Verification items for the finished model (mm, model axes). A direction names the side the tool comes from. Round coordinates to 2 decimals unless told otherwise and drop trailing zeros. Loops run counter-clockwise (first coordinate to the right, second up) from the corner with the lowest first, then second, coordinate; pieces in that order, holes last. Notation, with made-up numbers: (20, 23) -> (28, 23) arc R21 cw to (28, 53) -> close; hole circle Ø3 at (62.5, 19.25). An arc over 180 degrees is marked (long way). Write item = value, one per line.
```python
from build123d import *

# Parameters (mm, degrees)
SKETCH_1_R                = 33
SKETCH_1_R_2              = 25
EXTRUDE_1_DEPTH           = 8
SKETCH_3_W                = 6
SKETCH_3_H                = 75.065219084
CUT_EXTRUDE_1_DEPTH       = 4
CUT_EXTRUDE_1_DRAFT       = -1
HOLE_WIZARD_1_D           = 10
HOLE_WIZARD_1_CBORE_D     = 15.2
HOLE_WIZARD_1_CBORE_DEPTH = 4


with BuildPart() as part:
    # 草图1 → 凸台-拉伸1 (new body)
    # profile 1 of 2: a face of its own
    with BuildSketch(Plane.XY):
        Circle(SKETCH_1_R)
        Circle(SKETCH_1_R_2, mode=Mode.SUBTRACT)
    # profile 2 of 2: a face of its own
    with BuildSketch(Plane.XY):
        with BuildLine():
            Line((39.646094734, 37.429095265), (-3.509900495, 32.8128115))
            ThreePointArc((-3.509900495, 32.8128115), (22.058708979, 24.544110458), (33, 0))
            ThreePointArc((33, 0), (28.248342415, -17.059635132), (15.361748435, -29.206449374))
            ThreePointArc((15.361748435, -29.206449374), (23.844645568, -28.056684557), (31.078097518, -32.63474919))
            ThreePointArc((31.078097518, -32.63474919), (37.364061613, -36.96690321), (44.997122438, -36.835428905))
            Line((44.997122438, -36.835428905), (71, -28))
            Line((71, -28), (71, 28))
            Line((71, 28), (44.997122438, 36.835428905))
            ThreePointArc((44.997122438, 36.835428905), (42.353950178, 37.42377389), (39.646094734, 37.429095265))
        make_face()
    extrude(amount=EXTRUDE_1_DEPTH)


with BuildPart() as cut_extrude_1_tool:
    # 草图3 → 切除-拉伸-薄壁1 (with draft: the straight prism first)
    with BuildSketch(Plane(origin=(0, 0, 0), x_dir=(-1, 0, 0), z_dir=(0, 0, -1))):
        with Locations((0, -0.589324586)):
            Rectangle(SKETCH_3_W, SKETCH_3_H)
    extrude(amount=-CUT_EXTRUDE_1_DEPTH)
    # 切除-拉伸-薄壁1: the draft: its side faces are tilted about the plane it starts from
    cut_extrude_1_sides = [cut_extrude_1_tool.faces().sort_by_distance(p)[0] for p in [
        (3, -0.589324586, 2),
        (0, -38.121934128, 2),
        (-3, -0.589324586, 2),
        (0, 36.943284956, 2),
    ]]
    draft(cut_extrude_1_sides, Plane(origin=(0, 0, 0), x_dir=(-1, 0, 0), z_dir=(0, 0, -1)), CUT_EXTRUDE_1_DRAFT)


with BuildPart() as part_1:
    add(part.part)

    # 切除-拉伸-薄壁1: cut by cut_extrude_1_tool
    add(cut_extrude_1_tool.part, mode=Mode.SUBTRACT)

    # 孔1 (through all)
    with Locations(Plane.XY.offset(8)):
        with Locations((40.975602497, 25), (40.975602497, -25)):
            CounterBoreHole(HOLE_WIZARD_1_D / 2, HOLE_WIZARD_1_CBORE_D / 2, HOLE_WIZARD_1_CBORE_DEPTH)


solid = part_1.part
```
(1) Sectioned sample at D-D, the plane x = 56. Record the cut outline in (y, z), and give its area (3 significant figures).
Filled sheet:
outline = (-33.1, 0) -> (33.1, 0) -> (33.1, 8) -> (-33.1, 8) -> close
area = 530 mm2
(2) Go/stop test with flat-tipped pins: pin 1 Ø4 at (x, z) = (43.5, 1) entering from +Y; pin 2 Ø13.5 at (x, y) = (40.98, -25) entering from +Z; pin 3 Ø3 at (x, y) = (0.5, -30.5) entering from -Z. Record where each tip stops, or that it passes through.
Filled sheet:
pin_1 = 37.49
pin_2 = 4
pin_3 = 4
(3) Material ranges on probe 1 along X at (y, z) = (0, 3.25); probe 2 along Y at (x, z) = (38.5, 5.5); probe 3 along X at (y, z) = (-26, 3), recorded low to high. Write a range as from..to.
Filled sheet:
probe_1 = -33..-25, 25..71
probe_2 = -37.25..-32.19, -17.81..17.81, 32.19..37.31
probe_3 = -20.32..-2.95, 2.95..36.08, 45.87..71
(4) Draft check along X on faces 3 (the face through (0, -29, 4)), 4 (the face through (58.181, 32.356, 3.944)), 5 (the face through (18.37, 35.153, 3.944)), 6 (the face through (-26, -2, 0)). Enter one of: released by +X, released by -X, zero draft, split by the parting line, or undercut.
Filled sheet:
face_3 = undercut
face_4 = released by +X
face_5 = released by -X
face_6 = zero draft
(5) Set-up check for faces 1 (the face through (45.06, 31.41, 6.03)), 2 (the face through (44, 1, 0)): record each of +Z, -Z, +X, -X, +Y, -Y from which the full face is reachable in a straight line by a thin tool's end or side.
Filled sheet:
face_1 = +Z
face_2 = -Z, +X, -X, +Y, -Y
(6) Sectioned sample at B-B, the plane y = 0. Record the cut outline in (x, z).
Filled sheet:
outline = (-33, 0) -> (-25, 0) -> (-25, 8) -> (-33, 8) -> close; (25, 0) -> (71, 0) -> (71, 8) -> (25, 8) -> close
(7) Sectioned sample at A-A, the plane z = 2.5. Record the cut outline in (x, y), and give its area (3 significant figures).
Filled sheet:
outline = (-3.51, 32.81) arc R33 ccw to (-2.96, -32.87) -> (-2.96, -24.82) arc R25 cw to (-2.96, 24.82) -> (-2.96, 32.87) -> close; (2.96, -32.87) arc R33 ccw to (15.36, -29.21) arc R12.5 cw to (31.08, -32.63) arc R12.5 ccw to (45, -36.84) -> (71, -28) -> (71, 28) -> (45, 36.84) arc R12.5 ccw to (39.65, 37.43) -> (2.96, 33.5) -> (2.96, 24.82) arc R25 cw to (2.96, -24.82) -> close; hole circle Ø10 at (40.98, -25); hole circle Ø10 at (40.98, 25)
area = 4,230 mm2
(8) Sectioned sample at C-C, the plane x = 0. Record the cut outline in (y, z).
Filled sheet:
outline = (-33, 4) -> (-25, 4) -> (-25, 8) -> (-33, 8) -> close; (25, 4) -> (33.19, 4) -> (33.19, 8) -> (25, 8) -> close
